Can you work these out from the model? Positions are in its coordinate system, mm. A direction names the side the tool comes from. Round coordinates to 2 decimals unless told otherwise and drop trailing zeros. Loops run counter-clockwise (first coordinate to the right, second up) from the corner with the lowest first, then second, coordinate; pieces in that order, holes last. Notation, with made-up numbers: M 74,60 L 78,60 A15 cw 78,83 Z; hole C 87,41.5 d10. An arc over 180 degrees is marked long. Return JSON: item names as keys, results as strings.
```python
from build123d import *

# Parameters (mm, degrees)
SKETCH1_R                                        = 5
BOSS_EXTRUDE1_DEPTH                              = 30
SKETCH2_W                                        = 160
SKETCH2_H                                        = 30
BOSS_EXTRUDE2_DEPTH                              = 10
RIB1_REACH                                       = 529.146
SKETCH5_WALL_W                                   = 1084.577110596
SKETCH5_WALL_H                                   = 10
RIB17_REACH                                      = 529.146
SKETCH7_WALL_W                                   = 1084.577110596
SKETCH7_WALL_H                                   = 10
CBORE_FOR_M4_HEX_HEAD_MACHINE_SCREW2_D           = 4.5
CBORE_FOR_M4_HEX_HEAD_MACHINE_SCREW2_CBORE_D     = 10.59
CBORE_FOR_M4_HEX_HEAD_MACHINE_SCREW2_CBORE_DEPTH = 3
MIRROR2_COPY_1_D                                 = 4.5
MIRROR2_COPY_1_CBORE_D                           = 10.59
MIRROR2_COPY_1_CBORE_DEPTH                       = 3
BOSS_EXTRUDE5_DEPTH                              = 90
CUT_EXTRUDE4_DEPTH                               = 100
CUT_EXTRUDE4_DEPTH_BACK                          = 100
CUT_EXTRUDE5_DEPTH                               = 8.65
CUT_EXTRUDE6_DEPTH                               = 8.65


with BuildPart() as part:
    # Sketch1 → Boss-Extrude1 (new body)
    with BuildSketch(Plane.XY):
        with BuildLine():
            Line((-7.071067812, 7.071067812), (75.857864376, 90))
            Line((75.857864376, 90), (375.857864376, 90))
            ThreePointArc((375.857864376, 90), (411.213203436, 75.355339059), (425.857864376, 40))
            Line((425.857864376, 40), (425.857864376, -260))
            Line((425.857864376, -260), (325.857864376, -360))
            Line((325.857864376, -360), (325.857864376, -410))
            Line((325.857864376, -410), (205.857864376, -400))
            Line((205.857864376, -400), (205.857864376, -380))
            Line((205.857864376, -380), (295.857864376, -380))
            Line((295.857864376, -380), (295.857864376, -300))
            Line((295.857864376, -300), (335.857864376, -260))
            Line((335.857864376, -260), (335.857864376, -60))
            ThreePointArc((335.857864376, -60), (321.213203436, -24.644660941), (285.857864376, -10))
            Line((285.857864376, -10), (0, -10))
            ThreePointArc((0, -10), (-9.238795325, -3.826834324), (-7.071067812, 7.071067812))
        make_face()
        Circle(SKETCH1_R, mode=Mode.SUBTRACT)
    extrude(amount=BOSS_EXTRUDE1_DEPTH)

    # Sketch2 → Boss-Extrude2 (add)
    with BuildSketch(Plane.XZ.offset(10)):
        with Locations((100, 45)):
            Rectangle(SKETCH2_W, SKETCH2_H)
        with Locations((100, 15)):
            Rectangle(SKETCH2_W, SKETCH2_H)
        with Locations((100, -15)):
            Rectangle(SKETCH2_W, SKETCH2_H)
    extrude(amount=BOSS_EXTRUDE2_DEPTH)

    # Sketch5 wall → Rib1 (add, up to next)
    with BuildSketch(Plane(origin=(100, 0, 40), x_dir=(0, -0.707106781187, 0.707106781187), z_dir=(0, 0.707106781187, 0.707106781187)), mode=Mode.PRIVATE) as rib1_sk1:
        Rectangle(SKETCH5_WALL_W, SKETCH5_WALL_H)
    rib1_tool1 = extrude(rib1_sk1.sketch, amount=-RIB1_REACH, mode=Mode.PRIVATE) - part.part
    add(rib1_tool1.solids().sort_by_distance((100, 0, 40))[0])

    # Sketch7 wall → Rib17 (add, up to next)
    with BuildSketch(Plane(origin=(100, 0, -10), x_dir=(0, -0.707106781187, -0.707106781187), z_dir=(0, -0.707106781187, 0.707106781187)), mode=Mode.PRIVATE) as rib17_sk1:
        Rectangle(SKETCH7_WALL_W, SKETCH7_WALL_H)
    rib17_tool1 = extrude(rib17_sk1.sketch, amount=RIB17_REACH, mode=Mode.PRIVATE) - part.part
    add(rib17_tool1.solids().sort_by_distance((100, 0, -10))[0])

    # CBORE for M4 Hex Head Machine Screw2 (through all)
    with Locations(Plane(origin=(0, -10, 0), x_dir=(1, 0, 0), z_dir=(0, 1, 0))):
        with Locations((130, -48.5), (150, -48.5), (170, -48.5)):
            cbore_for_m4_hex_head_machine_screw2 = CounterBoreHole(CBORE_FOR_M4_HEX_HEAD_MACHINE_SCREW2_D / 2, CBORE_FOR_M4_HEX_HEAD_MACHINE_SCREW2_CBORE_D / 2, CBORE_FOR_M4_HEX_HEAD_MACHINE_SCREW2_CBORE_DEPTH)

    # Mirror1: CBORE for M4 Hex Head Machine Screw2 across plane
    add(cbore_for_m4_hex_head_machine_screw2.mirror(Plane(origin=(100, 0, 0), x_dir=(0, 0, 1), z_dir=(1, 0, 0))), mode=Mode.SUBTRACT)

    # Mirror2: CBORE for M4 Hex Head Machine Screw2 across plane
    add(cbore_for_m4_hex_head_machine_screw2.mirror(Plane.XY.offset(16)), mode=Mode.SUBTRACT)

    # Mirror2 copy 1 (through all)
    with Locations(Plane(origin=(200, -10, 32), x_dir=(-1, 0, 0), z_dir=(0, 1, 0))):
        with Locations((130, -48.5), (150, -48.5), (170, -48.5)):
            CounterBoreHole(MIRROR2_COPY_1_D / 2, MIRROR2_COPY_1_CBORE_D / 2, MIRROR2_COPY_1_CBORE_DEPTH)

    # Sketch19 → Boss-Extrude5 (add)
    with BuildSketch(Plane.ZY.offset(-295.857864376)):
        with BuildLine():
            Line((-23.890872965, -394.024153256), (-16.819805153, -401.095221068))
            ThreePointArc((-16.819805153, -401.095221068), (15, -387.915026221), (46.819805153, -401.095221068))
            Line((46.819805153, -401.095221068), (53.890872965, -394.024153256))
            ThreePointArc((53.890872965, -394.024153256), (15, -377.915026221), (-23.890872965, -394.024153256))
        make_face()
    extrude(amount=BOSS_EXTRUDE5_DEPTH)

    # Sketch20 → Cut-Extrude4 (cut, two sides)
    with BuildSketch(Plane(origin=(-31.683738866, -380.204866396, 0), x_dir=(0.9965457582448797, -0.08304547985374006, 0), z_dir=(-0.08304547985374006, -0.9965457582448797, 0))) as cut_extrude4_sk:
        Polygon((228.178842993, -32.182148517), (344.185851358, -32.182148517), (238.364973487, 0), (228.178842993, 3.097796682), align=None)
        Polygon((238.364973487, 30), (346.499317462, 62.242718318), (228.178842993, 62.242718318), (228.178842993, 26.962773119), align=None)
    extrude(amount=CUT_EXTRUDE4_DEPTH, mode=Mode.SUBTRACT)
    extrude(cut_extrude4_sk.sketch, amount=-CUT_EXTRUDE4_DEPTH_BACK, mode=Mode.SUBTRACT)

    # Sketch21 → Cut-Extrude5 (cut)
    with BuildSketch(Plane.XY.offset(30)):
        with BuildLine():
            Line((206.65047943, -390.48861935), (205.857864376, -390.48861935))
            Line((205.857864376, -390.48861935), (205.857864376, -400))
            Line((205.857864376, -400), (325.857864376, -410))
            Line((325.857864376, -410), (325.857864376, -360))
            Line((325.857864376, -360), (425.857864376, -260))
            Line((425.857864376, -260), (425.857864376, 40))
            ThreePointArc((425.857864376, 40), (411.213203436, 75.355339059), (375.857864376, 90))
            Line((375.857864376, 90), (75.857864376, 90))
            Line((75.857864376, 90), (-7.071067812, 7.071067812))
            ThreePointArc((-7.071067812, 7.071067812), (-9.238795325, -3.826834324), (0, -10))
            Line((0, -10), (20, -10))
            Line((20, -10), (95, -10))
            Line((95, -10), (95, 10))
            Line((95, 10), (105, 10))
            Line((105, 10), (105, -10))
            Line((105, -10), (180, -10))
            Line((180, -10), (285.857864376, -10))
            ThreePointArc((285.857864376, -10), (321.213203436, -24.644660941), (335.857864376, -60))
            Line((335.857864376, -60), (335.857864376, -260))
            Line((335.857864376, -260), (295.857864376, -300))
            Line((295.857864376, -300), (295.857864376, -380))
            Line((295.857864376, -380), (295.857864376, -390.48861935))
            Line((295.857864376, -390.48861935), (206.65047943, -390.48861935))
        make_face()
    extrude(amount=-CUT_EXTRUDE5_DEPTH, mode=Mode.SUBTRACT)

    # Sketch22 → Cut-Extrude6 (cut)
    with BuildSketch(Plane(origin=(0, 0, 0), x_dir=(-1, 0, 0), z_dir=(0, 0, -1))):
        with BuildLine():
            Line((-206.65047943, -390.48861935), (-205.857864376, -390.48861935))
            Line((-205.857864376, -390.48861935), (-205.857864376, -400))
            Line((-205.857864376, -400), (-325.857864376, -410))
            Line((-325.857864376, -410), (-325.857864376, -360))
            Line((-325.857864376, -360), (-425.857864376, -260))
            Line((-425.857864376, -260), (-425.857864376, 40))
            ThreePointArc((-425.857864376, 40), (-411.213203436, 75.355339059), (-375.857864376, 90))
            Line((-375.857864376, 90), (-75.857864376, 90))
            Line((-75.857864376, 90), (7.071067812, 7.071067812))
            ThreePointArc((7.071067812, 7.071067812), (9.238795325, -3.826834324), (0, -10))
            Line((0, -10), (-20, -10))
            Line((-20, -10), (-95, -10))
            Line((-95, -10), (-95, 10))
            Line((-95, 10), (-105, 10))
            Line((-105, 10), (-105, -10))
            Line((-105, -10), (-180, -10))
            Line((-180, -10), (-285.857864376, -10))
            ThreePointArc((-285.857864376, -10), (-321.213203436, -24.644660941), (-335.857864376, -60))
            Line((-335.857864376, -60), (-335.857864376, -260))
            Line((-335.857864376, -260), (-295.857864376, -300))
            Line((-295.857864376, -300), (-295.857864376, -380))
            Line((-295.857864376, -380), (-295.857864376, -390.48861935))
            Line((-295.857864376, -390.48861935), (-206.65047943, -390.48861935))
        make_face()
    extrude(amount=-CUT_EXTRUDE6_DEPTH, mode=Mode.SUBTRACT)


solid = part.part
```
Q1. Suppose I cut it at C-C, the plane y = 34. Please give me the cut outline in (x, z).
Results:
{"outline": "M 19.86,8.65 L 425.86,8.65 L 425.86,21.35 L 19.86,21.35 Z"}
Q2. Suppose I cut it at B-B, the plane y = -232.5. Please give me the cut outline in (x, z).
Results:
{"outline": "M 335.86,8.65 L 425.86,8.65 L 425.86,21.35 L 335.86,21.35 Z"}
Q3. On a 3-axis mill with a long thin cutter (end or side, diameter ignored), from which of +Z, -Z, +X, -X, +Y, -Y can I reach the whole of each face in a straight line? I mean faces 4 (the flat face through (10, -10, 15)), 5 (the flat face through (295.858, -390, 37)), 6 (the flat face through (335.858, -161, 15)), 7 (the flat face through (95, -2, 33)), 8 (the cylindrical face through (75.29, -11.48, -16.27)). Say none if no direction works.
Results:
{"face 4": "+Z, -Z, -X, -Y", "face 5": "+Z, +X, +Y, -Y", "face 6": "+Z, -Z, -X", "face 7": "+Z, -X, +Y", "face 8": "+Y"}
Q4. Suppose I cut it at A-A, the plane z = 14.5. Please give me the cut outline in (x, y), plus the area to 3 significant figures.
Results:
{"outline": "M -7.07,7.07 A10 ccw 0,-10 L 20,-10 L 20,-20 L 180,-20 L 180,-10 L 285.86,-10 A50 cw 335.86,-60 L 335.86,-260 L 295.86,-300 L 295.86,-377.92 L 205.86,-377.92 L 205.86,-400 L 325.86,-410 L 325.86,-360 L 425.86,-260 L 425.86,40 A50 ccw 375.86,90 L 75.86,90 Z; hole C 0,0 d10", "area": "74,900 mm2"}
Q5. Thinking about a two-plate mould opening in Y: for faces 1 (the cylindrical face through (164.71, -11.48, -16.27)), 2 (the flat face through (130, -13, -19)), 3 (the flat face through (315.58, -280.28, 14.91)), which applies, pulls with the +Y half, pulls with the -Y half, needs draft (parallel to the pull), parting line crosses it, or undercut?
Results:
{"face 1": "needs draft", "face 2": "pulls with the +Y half", "face 3": "undercut"}
Q6. If I drill on line 1 along Z through (x, y) = (30, -16.5); line 2 along Z through (x, y) = (50, -11.3) (3 decimals); line 3 along X through (y, z) = (-5, -9.5), over which ranges is the centre line in solid material (lowest first)?
Results:
{"line 1": "z = -30 to -18.75, -14.25 to 46.25, 50.75 to 60", "line 2": "z = -30 to -21.795, -11.205 to 43.205, 53.795 to 60", "line 3": "x = 95 to 105"}
Q7. I'm going to push flat-ended pins straight in: pin 1 Ø5 at (y, z) = (-14.5, 23.5) entering from -X; pin 2 Ø5 at (x, z) = (30, 48.5) entering from -Y; pin 3 Ø10 at (x, y) = (331, -99.5) entering from -Z; pin 4 Ø3.5 at (x, z) = (150, -16.5) entering from -Y. Where does each tip first touch, or does it pass through?
Results:
{"pin 1": "stops at x = 20", "pin 2": "stops at y = -20", "pin 3": "stops at z = 8.65", "pin 4": "passes through"}
